Part print with two shaded views. Sizes in mm from the minimum x, y, z corner. Round coordinates to 2 decimals unless told otherwise and drop trailing zeros. Write each loop counter-clockwise with the first axis right and the second up, starting at its lowest first coordinate (ties: lowest second). Pieces come first, ordered by that corner, then holes.
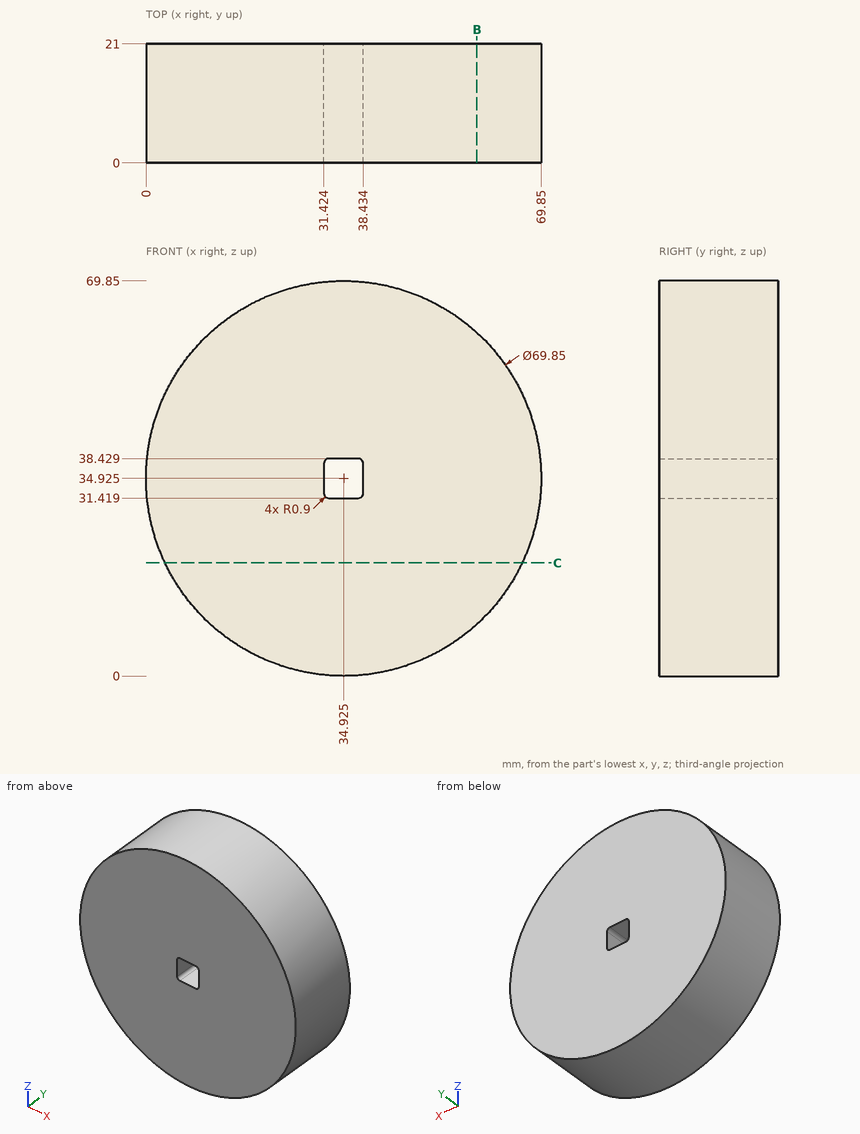
Q1. Cut at B-B on x = 58.5. Write the cut outline in (y, z).
Values follow:
outline: (0, 9.16) - (21, 9.16) - (21, 60.69) - (0, 60.69) - close
Q2. Drop flat-ended pins along their axis: pin 1 (4 mm diameter, centred on y = 8.5, z = 35.5, fed in from -X); pin 2 (6 mm diameter, centred on y = 5, z = 40.5, fed in from -X) (3 decimals); pin 3 (1 mm diameter, centred on x = 40, y = 9, fed in from -Z); pin 4 (5.5 mm diameter, centred on x = 34, y = 12, fed in from -Z). Give the stop position or say it passes through.
Values follow:
pin 1: stops at x = 0
pin 2: stops at x = 0.095
pin 3: stops at z = 0.3
pin 4: stops at z = 0
Q3. Wall check: L1, parallel to Z at x = 32.5, y = 4 (1 decimal); L2, parallel to Z at x = 17, y = 3.25; L3, parallel to X at y = 6, z = 45.5. Give the ranges that are in metal, low to high.
Values follow:
L1: z = 0.1 to 31.4, 38.4 to 69.8
L2: z = 4.95 to 64.9
L3: x = 1.64 to 68.21
Q4. Cut at C-C on z = 20. Write the cut outline in (x, y).
Values follow:
outline: (3.35, 0) - (66.5, 0) - (66.5, 21) - (3.35, 21) - close
